from build123d import *

# Parameters (mm, degrees)
EXTRUDE_THIN1_DEPTH = 584.2
SKETCH3_W           = 15.24
SKETCH3_H           = 3.302
CUT_EXTRUDE1_DEPTH  = 614.413196966


with BuildPart() as part:
    # Sketch2 → Extrude-Thin1 (new body)
    with BuildSketch(Plane(origin=(0, 0, 0), x_dir=(0, 0, -1), z_dir=(1, 0, 0))):
        with BuildLine():
            ThreePointArc((100.125623552, -111.716090426), (136.978732363, -61.175585258), (150.01875, 0))
            Line((150.01875, 0), (148.43125, 0))
            ThreePointArc((148.43125, 0), (135.529221968, -60.528224568), (99.066093144, -110.533909574))
            Line((99.066093144, -110.533909574), (100.125623552, -111.716090426))
        make_face()
    extrude(amount=EXTRUDE_THIN1_DEPTH)

    # Sketch3 → Cut-Extrude1 (cut, through all)
    with BuildSketch(Plane.XY):
        with Locations((7.62, -92.372909574)):
            Rectangle(SKETCH3_W, SKETCH3_H)
        with Locations((576.58, -92.372909574)):
            Rectangle(SKETCH3_W, SKETCH3_H)
    extrude(amount=-CUT_EXTRUDE1_DEPTH, mode=Mode.SUBTRACT)


solid = part.part
Model file for the job. Use its own axes, mm. Round coordinates to 2 decimals unless told otherwise and drop trailing zeros. Order: outer loops, then holes, each group sorted by start corner. A loop starts at its lowest first (then second) coordinate and runs counter-clockwise, first axis right, second up.
(1) Band-saw the part on B-B (y = -76.5). List the corners of the cut face in (x, z).
(2) Drill centre lines: line 1 (Y direction, x = 210, z = -130); line 2 (Z direction, x = 338.5, y = -27); line 3 (Y direction, x = 80.5, z = -126). Where is each one in solid material? Low to high.
(3) Band-saw the part on A-A (x = 426). List the corners of the cut face in (y, z).
(4) Pin check, flat tips, straight feed: pin 1 (4 mm diameter, centred on x = 268, y = -77.5, fed in from +Z); pin 2 (12 mm diameter, centred on x = 514.5, y = -29, fed in from -Z); pin 3 (1.5 mm diameter, centred on x = 422, z = -105.5, fed in from -Y). Stop position of each tip, or through.
Verdict:
1. outline: (0, -129.05) - (584.2, -129.05) - (584.2, -127.2) - (0, -127.2) - close
2. line 1: y = -74.87 to -71.64
2. line 2: z = -147.57 to -145.95
2. line 3: y = -81.42 to -78.46
3. outline: (-111.72, -100.13) arc R150.02 ccw to (0, -150.02) - (0, -148.43) arc R148.43 cw to (-110.53, -99.07) - close
4. pin 1: stops at z = -125.35
4. pin 2: stops at z = -148.25
4. pin 3: stops at y = -107.39
